```python
from build123d import *

# Parameters (mm, degrees)
SKETCH1_W           = 93
SKETCH1_H           = 100
BOSS_EXTRUDE2_DEPTH = 6.3
SKETCH3_W           = 35
SKETCH3_H           = 100
BOSS_EXTRUDE3_DEPTH = 5
SKETCH4_W           = 11.3
SKETCH4_H           = 15
BOSS_EXTRUDE4_DEPTH = 24
SKETCH5_R           = 2
CUT_EXTRUDE1_DEPTH  = 50
SKETCH6_R           = 8.115
CUT_EXTRUDE2_DEPTH  = 50
SKETCH7_R           = 11
CUT_EXTRUDE3_DEPTH  = 50
EXTRUDE_THIN1_START = -5.3
SKETCH7_2_R         = 11
SKETCH7_2_R_2       = 9
EXTRUDE_THIN1_DEPTH = 1
EXTRUDE_THIN2_START = -10.3
SKETCH6_2_R         = 8.115
SKETCH6_2_R_2       = 6.115
EXTRUDE_THIN2_DEPTH = 1


with BuildPart() as part:
    # Sketch1 → Boss-Extrude2 (new body)
    with BuildSketch(Plane.XY):
        with Locations((-29.68705036, 14.928057554)):
            Rectangle(SKETCH1_W, SKETCH1_H)
    extrude(amount=BOSS_EXTRUDE2_DEPTH)

    # Sketch3 → Boss-Extrude3 (add)
    with BuildSketch(Plane(origin=(0, 0, 0), x_dir=(-1, 0, 0), z_dir=(0, 0, -1))):
        with Locations((0.68705036, 14.928057554)):
            Rectangle(SKETCH3_W, SKETCH3_H)
    extrude(amount=BOSS_EXTRUDE3_DEPTH)

    # Sketch4 → Boss-Extrude4 (add)
    with BuildSketch(Plane(origin=(16.81294964, 0, 0), x_dir=(0, 0, -1), z_dir=(1, 0, 0))):
        with Locations((-0.65, -21.271942446)):
            Rectangle(SKETCH4_W, SKETCH4_H)
    extrude(amount=BOSS_EXTRUDE4_DEPTH)

    # Sketch5 → Cut-Extrude1 (cut)
    with BuildSketch(Plane(origin=(0, -13.771942446, 0), x_dir=(1, 0, 0), z_dir=(0, 1, 0))):
        with Locations(Location((28.81294964, -0.8, 0), (0, 0, 180))):
            Circle(SKETCH5_R)
    extrude(amount=-CUT_EXTRUDE1_DEPTH, mode=Mode.SUBTRACT)

    # Sketch6 → Cut-Extrude2 (cut)
    with BuildSketch(Plane(origin=(0, 0, -5), x_dir=(-1, 0, 0), z_dir=(0, 0, -1))):
        with Locations((-1.81294964, -15.071942446)):
            Circle(SKETCH6_R)
    extrude(amount=-CUT_EXTRUDE2_DEPTH, mode=Mode.SUBTRACT)

    # Sketch7 → Cut-Extrude3 (cut)
    with BuildSketch(Plane(origin=(0, 0, 0), x_dir=(-1, 0, 0), z_dir=(0, 0, -1))):
        with Locations((58.18705036, 44.928057554)):
            Circle(SKETCH7_R)
    extrude(amount=-CUT_EXTRUDE3_DEPTH, mode=Mode.SUBTRACT)

    # Sketch7<2> → Extrude-Thin1 (add)
    with BuildSketch(Plane(origin=(0, 0, 0), x_dir=(-1, 0, 0), z_dir=(0, 0, -1)).offset(EXTRUDE_THIN1_START)):
        with Locations((58.18705036, 44.928057554)):
            Circle(SKETCH7_2_R)
        with Locations((58.18705036, 44.928057554)):
            Circle(SKETCH7_2_R_2, mode=Mode.SUBTRACT)
    extrude(amount=-EXTRUDE_THIN1_DEPTH)

    # Sketch6<2> → Extrude-Thin2 (add)
    with BuildSketch(Plane(origin=(0, 0, -5), x_dir=(-1, 0, 0), z_dir=(0, 0, -1)).offset(EXTRUDE_THIN2_START)):
        with Locations((-1.81294964, -15.071942446)):
            Circle(SKETCH6_2_R)
        with Locations((-1.81294964, -15.071942446)):
            Circle(SKETCH6_2_R_2, mode=Mode.SUBTRACT)
    extrude(amount=-EXTRUDE_THIN2_DEPTH)


solid = part.part
```
The listing builds one solid part. Answer for the finished solid, in the listing's coordinates (mm). A direction names the side the tool comes from. Give positions to 0.01 mm unless a question says otherwise; leave off trailing zeros. Order: outer loops, then holes, each group sorted by start corner. A loop starts at its lowest first (then second) coordinate and runs counter-clockwise, first axis right, second up. Notation, with made-up numbers: M 78,-7 L 96,-7 A32 cw 96,30 Z; hole C 46.25,39.25 d7. An arc over 180 degrees is marked long. Put each result on its own line as item: value. Start each with the question number.
Item 1: The part is cut by section C-C, the plane y = -1.5. Determine the outline of the cut face in (x, z), and give its area (3 significant figures).
Item 2: Flat-ended cylindrical pins translate along their axes: P1, Ø5, axis at y = 21.5, z = -3.5, coming from the +X side; P2, Ø17.5, axis at x = -47.5, y = 15.5, coming from the -Z side; P3, Ø14, axis at x = 1.81, y = -15.07, coming from the -Z side; P4, Ø5, axis at x = 0, y = -15.5, coming from the -Z side. Find the tip coordinate at first contact, or state that the pin passes through.
Item 3: Find the intervals of material crossed by line 1 along Z through (x, y) = (-26.5, 17); line 2 along X through (y, z) = (61, 2.5); line 3 along Y through (x, z) = (32.5, -0.5), in increasing order.
Item 4: The part is cut by section A-A, the plane x = 4. Determine the outline of the cut face in (y, z), and give its area (3 significant figures).
Item 5: The part is cut by section D-D, the plane x = -55.5. Determine the outline of the cut face in (y, z).
Item 6: For a pull along X with two mould halves and no side action, classify faces 6 (the face through (-18.187, 14, -2)), 7 (the face through (3.14, -21.04, 5.79)), 8 (the face through (-19, 64.928, 2)) as +X half, -X half, draft (parallel to the pull), parting line (faces both ways), or undercut.
Item 7: Which of the six approach directions +Z, -Z, +X, -X, +Y, -Y give full straight-line access (tool end or side, diameter ignored) to faces 1 (the face through (3.572, -22.994, 0.078)), 2 (the face through (40.813, -21, 1)), 3 (the face through (29, -28.772, 3)), 4 (the face through (-48, 16, 0)), 5 (the face through (29, -13.772, 3))?
Item 8: The part is cut by section B-B, the plane y = 38.5. Determine the outline of the cut face in (x, z), and give its area (3 significant figures).
Answer key:
1. outline: M -76.19,0 L -18.19,0 L -18.19,-5 L 16.81,-5 L 16.81,6.3 L -76.19,6.3 Z
1. area: 761 mm²
2. P1: stops at x = 16.81
2. P2: stops at z = 0
2. P3: stops at z = 5.3
2. P4: passes through
3. line 1: z = 0 to 6.3
3. line 2: x = -76.19 to 16.81
3. line 3: y = -28.77 to -13.77
4. outline: M -35.07,-5 L -22.89,-5 L -22.89,5.3 L -20.78,5.3 L -20.78,6.3 L -35.07,6.3 Z; M -9.36,5.3 L -7.26,5.3 L -7.26,-5 L 64.93,-5 L 64.93,6.3 L -9.36,6.3 Z
4. area: 958 mm²
5. outline: M -35.07,0 L 34.26,0 L 34.26,5.3 L 36.34,5.3 L 36.34,6.3 L -35.07,6.3 Z; M 53.52,5.3 L 55.59,5.3 L 55.59,0 L 64.93,0 L 64.93,6.3 L 53.52,6.3 Z
6. face 6: -X half
6. face 7: undercut
6. face 8: draft
7. face 1: -Z
7. face 2: +Z, -Z, +X, +Y, -Y
7. face 3: +Z, -Z, +X, -Y
7. face 4: -Z, -X, +Y, -Y
7. face 5: +Z, -Z, +X, +Y
8. outline: M -76.19,0 L -67.11,0 L -67.11,5.3 L -64.49,5.3 L -64.49,6.3 L -76.19,6.3 Z; M -51.89,5.3 L -49.26,5.3 L -49.26,0 L -18.19,0 L -18.19,-5 L 16.81,-5 L 16.81,6.3 L -51.89,6.3 Z
8. area: 654 mm²
